```python
from build123d import *

# Parameters (mm, degrees)
ESQUISSE1_W             = 25.8
ESQUISSE1_H             = 32.4
BOSS_EXTRU_1_DEPTH      = 10
ESQUISSE2_W             = 25.8
ESQUISSE2_H             = 12
BOSS_EXTRU_2_DEPTH      = 29
ESQUISSE3_R             = 2.75
ENL_V_MAT_EXTRU_1_DEPTH = 3
ESQUISSE4_R             = 1.75
ENL_V_MAT_EXTRU_2_DEPTH = 7
ESQUISSE5_W             = 22
ESQUISSE5_H             = 12
BOSS_EXTRU_3_DEPTH      = 12.08
CONG_1_R                = 5
ENL_V_START             = -12
ESQUISSE6_R             = 2.5
ENL_V_MAT_EXTRU_3_DEPTH = 12
ESQUISSE7_R             = 3.6
ENL_V_MAT_EXTRU_4_DEPTH = 4
ESQUISSE8_W             = 2.91
ESQUISSE8_H             = 5.5
ENL_V_MAT_EXTRU_5_DEPTH = 3


with BuildPart() as part:
    # Esquisse1 → Boss.-Extru.1 (new body)
    with BuildSketch(Plane.XY):
        with Locations((2.080747766, -4.221428571)):
            Rectangle(ESQUISSE1_W, ESQUISSE1_H)
    extrude(amount=BOSS_EXTRU_1_DEPTH)

    # Esquisse2 → Boss.-Extru.2 (add)
    with BuildSketch(Plane.XY.offset(10)):
        with Locations((2.080747766, -4.221428571)):
            Rectangle(ESQUISSE2_W, ESQUISSE2_H)
    extrude(amount=BOSS_EXTRU_2_DEPTH)

    # Esquisse3 → Enlèv. mat.-Extru.1 (cut)
    with BuildSketch(Plane.XY.offset(10)):
        with Locations((12.070747766, 5.778571429)):
            Circle(ESQUISSE3_R)
        with Locations((-7.909252234, 5.778571429)):
            Circle(ESQUISSE3_R)
        with Locations((-7.909252234, -14.221428571)):
            Circle(ESQUISSE3_R)
        with Locations((12.070747766, -14.221428571)):
            Circle(ESQUISSE3_R)
    extrude(amount=-ENL_V_MAT_EXTRU_1_DEPTH, mode=Mode.SUBTRACT)

    # Esquisse4 → Enlèv. mat.-Extru.2 (cut)
    with BuildSketch(Plane.XY.offset(7)):
        with Locations((12.070747766, 5.778571429)):
            Circle(ESQUISSE4_R)
        with Locations((-7.909252234, 5.778571429)):
            Circle(ESQUISSE4_R)
        with Locations((12.070747766, -14.221428571)):
            Circle(ESQUISSE4_R)
        with Locations((-7.909252234, -14.221428571)):
            Circle(ESQUISSE4_R)
    extrude(amount=-ENL_V_MAT_EXTRU_2_DEPTH, mode=Mode.SUBTRACT)

    # Esquisse5 → Boss.-Extru.3 (add)
    with BuildSketch(Plane.ZY.offset(10.819252234)):
        with Locations((28, -4.221428571)):
            Rectangle(ESQUISSE5_W, ESQUISSE5_H)
    extrude(amount=BOSS_EXTRU_3_DEPTH)

    # Congé1
    cong_1_edges = [part.edges().sort_by_distance(p)[0] for p in [
        (-22.899252234, -4.221428571, 17),
    ]]
    fillet(cong_1_edges, radius=CONG_1_R)

    # Esquisse6 → Enlèv. mat.-Extru.3 (cut)
    with BuildSketch(Plane.XZ.offset(10.221428571).offset(ENL_V_START)):
        with Locations((-16.899252234, 23)):
            Circle(ESQUISSE6_R)
    extrude(amount=ENL_V_MAT_EXTRU_3_DEPTH, mode=Mode.SUBTRACT)

    # Esquisse7 → Enlèv. mat.-Extru.4 (cut)
    with BuildSketch(Plane(origin=(0, 1.778571429, 0), x_dir=(1, 0, 0), z_dir=(0, 1, 0))):
        with Locations(Location((-16.899252234, -23, 0), (0, 0, 270))):
            Circle(ESQUISSE7_R)
    extrude(amount=-ENL_V_MAT_EXTRU_4_DEPTH, mode=Mode.SUBTRACT)

    # Esquisse8 → Enlèv. mat.-Extru.5 (cut)
    with BuildSketch(Plane.XY.offset(10)):
        with Locations((13.525747766, -14.221428571)):
            Rectangle(ESQUISSE8_W, ESQUISSE8_H)
        with Locations((13.525747766, 5.778571429)):
            Rectangle(ESQUISSE8_W, ESQUISSE8_H)
        with Locations((-9.364252234, 5.778571429)):
            Rectangle(ESQUISSE8_W, ESQUISSE8_H)
        with Locations((-9.364252234, -14.221428571)):
            Rectangle(ESQUISSE8_W, ESQUISSE8_H)
    extrude(amount=-ENL_V_MAT_EXTRU_5_DEPTH, mode=Mode.SUBTRACT)


solid = part.part
```
Could you check a few things on this model? Use its own coordinates, in mm. A direction names the side the tool comes from. Give positions to 0.01 mm unless a question says otherwise; leave off trailing zeros. Loops run counter-clockwise (first coordinate to the right, second up) from the corner with the lowest first, then second, coordinate; pieces in that order, holes last. Notation, with made-up numbers: (56.25, -6) -> (62.25, -6) arc R11 cw to (62.25, 9) -> close; hole circle Ø6 at (61.25, 57.5). An arc over 180 degrees is marked (long way). Put each result on its own line as item: value.
(1) Imagine slicing it at B-B on x = -18.5. Write out the boundary of the cut face in (y, z).
Computed:
outline: (-10.22, 17.04) -> (1.78, 17.04) -> (1.78, 19.78) -> (-2.22, 19.78) -> (-2.22, 21.08) -> (-10.22, 21.08) -> close; (-10.22, 24.92) -> (-2.22, 24.92) -> (-2.22, 26.22) -> (1.78, 26.22) -> (1.78, 39) -> (-10.22, 39) -> close
(2) For faces 1 (the face through (2, 7, 10)), 2 (the face through (-5.16, 5.72, 8.52)), 3 (the face through (-10.819, -4, 6)), 4 (the face through (14, -16.971, 9)), which set-ups out of +Z, -Z, +X, -X, +Y, -Y let a thin tool reach every point of the face, with its end or its side?
Computed:
face 1: +Z, +X, -X, +Y
face 2: +Z, -X
face 3: -Z, -X, +Y, -Y
face 4: +Z, +X
(3) Please list where these lines run through material, in increasing order: probe 1 along X at (y, z) = (-0.35, 23); probe 2 along Y at (x, z) = (-3, 15); probe 3 along Z at (x, y) = (-10.5, 4.5). Write a range as [from, to].
Computed:
probe 1: [-22.9, -20.5], [-13.3, 14.98]
probe 2: [-10.22, 1.78]
probe 3: [0, 7]
(4) Thinking about a two-plate mould opening in Z: for faces 5 (the face through (-14, -2.221, 24)), 6 (the face through (-10, -14, 7)), 7 (the face through (14.981, -4, 15)), which applies, pulls with the +Z half, pulls with the -Z half, needs draft (parallel to the pull), parting line crosses it, or undercut?
Computed:
face 5: undercut
face 6: pulls with the +Z half
face 7: needs draft
(5) Imagine slicing it at A-A on z = 23. Write out the boundary of the cut face in (x, y).
Computed:
outline: (-22.9, -10.22) -> (-19.4, -10.22) -> (-19.4, -2.22) -> (-20.5, -2.22) -> (-20.5, 1.78) -> (-22.9, 1.78) -> close; (-14.4, -10.22) -> (14.98, -10.22) -> (14.98, 1.78) -> (-13.3, 1.78) -> (-13.3, -2.22) -> (-14.4, -2.22) -> close
(6) Imagine slicing it at C-C on y = -7.5. Write out the boundary of the cut face in (x, z).
Computed:
outline: (-22.9, 22) arc R5 ccw to (-17.9, 17) -> (-10.82, 17) -> (-10.82, 0) -> (14.98, 0) -> (14.98, 39) -> (-22.9, 39) -> close; hole circle Ø5 at (-16.9, 23)
(7) I'm going to push flat-ended pins straight in: pin 1 Ø11.5 at (x, z) = (-16.9, 23) entering from +Y; pin 2 Ø4 at (x, z) = (-12.5, 20) entering from -Y; pin 3 Ø3 at (y, z) = (3.5, 14) entering from +X; pin 4 Ø1.6 at (x, y) = (13, -13.5) entering from +Z. Where does each tip first touch, or does it pass through?
Computed:
pin 1: y = 1.78
pin 2: y = -10.22
pin 3: through
pin 4: z = 7
(8) Imagine slicing it at D-D on x = -9. Write out the boundary of the cut face in (y, z).
Computed:
outline: (-20.42, 0) -> (-15.59, 0) -> (-15.59, 7) -> (-16.97, 7) -> (-16.97, 10) -> (-20.42, 10) -> close; (-12.85, 0) -> (4.41, 0) -> (4.41, 7) -> (3.03, 7) -> (3.03, 10) -> (1.78, 10) -> (1.78, 39) -> (-10.22, 39) -> (-10.22, 10) -> (-11.47, 10) -> (-11.47, 7) -> (-12.85, 7) -> close; (7.15, 0) -> (11.98, 0) -> (11.98, 10) -> (8.53, 10) -> (8.53, 7) -> (7.15, 7) -> close
